Autodesk Inventor part; units mm, degrees
ref_plane "YZ Plane" through (0, 0, 0) normal (1, 0, 0) x (0, 1, 0)
ref_plane "XZ Plane" through (0, 0, 0) normal (0, 1, 0) x (-1, 0, 0)
ref_plane "XY Plane" through (0, 0, 0) normal (0, 0, 1) x (1, 0, 0)
sketch "Sketch1" plane through (0, 0, 0) normal (0, 0, 1) x (1, 0, 0)
  circle A0 centre (0, 0) radius 16.5
  arc A1 (-19.8431, 22.5) -> (-22.5, 19.8431) centre (0, 0) ccw
  arc A2 (22.5, 19.8431) -> (19.8431, 22.5) centre (0, 0) ccw
  arc A3 (-22.5, -19.8431) -> (-19.8431, -22.5) centre (0, 0) ccw
  arc A4 (19.8431, -22.5) -> (22.5, -19.8431) centre (0, 0) ccw
  line L0 (-22.5, -15) -> (-19.5, -12)
  line L1 (-19.5, 12) -> (-22.5, 15)
  line L2 (-15, -22.5) -> (-12, -19.5)
  line L3 (12, -19.5) -> (15, -22.5)
  line L4 (22.5, -15) -> (19.5, -12)
  line L5 (19.5, 12) -> (22.5, 15)
  line L6 (-22.5, -19.8431) -> (-22.5, -15)
  line L7 (-22.5, 15) -> (-22.5, 19.8431)
  line L8 (19.8431, -22.5) -> (15, -22.5)
  line L9 (-15, -22.5) -> (-19.8431, -22.5)
  line L10 (22.5, 19.8431) -> (22.5, 15)
  line L11 (22.5, -15) -> (22.5, -19.8431)
  line L12 (19.5, 4) -> (22.5, 4)
  line L13 (22.5, 4) -> (22.5, 2)
  line L14 (22.5, 2) -> (21.5, 2)
  line L15 (21.5, 2) -> (21.5, 3)
  line L16 (21.5, 3) -> (19.5, 3)
  line L17 (19.5, -4) -> (22.5, -4)
  line L18 (22.5, -4) -> (22.5, -2)
  line L19 (22.5, -2) -> (21.5, -2)
  line L20 (21.5, -2) -> (21.5, -3)
  line L21 (21.5, -3) -> (19.5, -3)
  line L22 (4, -19.5) -> (4, -22.5)
  line L23 (4, -22.5) -> (2, -22.5)
  line L24 (2, -22.5) -> (2, -21.5)
  line L25 (2, -21.5) -> (3, -21.5)
  line L26 (3, -21.5) -> (3, -19.5)
  line L27 (-3, -19.5) -> (-3, -21.5)
  line L28 (-3, -21.5) -> (-2, -21.5)
  line L29 (-2, -21.5) -> (-2, -22.5)
  line L30 (-2, -22.5) -> (-4, -22.5)
  line L31 (-4, -22.5) -> (-4, -19.5)
  line L32 (-19.5, -4) -> (-22.5, -4)
  line L33 (-22.5, -4) -> (-22.5, -2)
  line L34 (-22.5, -2) -> (-21.5, -2)
  line L35 (-21.5, -2) -> (-21.5, -3)
  line L36 (-21.5, -3) -> (-19.5, -3)
  line L37 (-19.5, 4) -> (-22.5, 4)
  line L38 (-22.5, 4) -> (-22.5, 2)
  line L39 (-22.5, 2) -> (-21.5, 2)
  line L40 (-21.5, 2) -> (-21.5, 3)
  line L41 (-21.5, 3) -> (-19.5, 3)
  line L42 (-12, -19.5) -> (-4, -19.5)
  line L43 (-3, -19.5) -> (3, -19.5)
  line L44 (4, -19.5) -> (12, -19.5)
  line L45 (-19.5, -12) -> (-19.5, -4)
  line L46 (-19.5, -3) -> (-19.5, 3)
  line L47 (-19.5, 4) -> (-19.5, 12)
  line L48 (19.5, -12) -> (19.5, -4)
  line L49 (19.5, -3) -> (19.5, 3)
  line L50 (19.5, 4) -> (19.5, 12)
  line L51 (-7.3937, 22.5) -> (-7, 27)
  line L52 (-7, 27) -> (7, 27)
  line L53 (7, 27) -> (7.3937, 22.5)
  arc A5 (-11.75, 20.9337) -> (-8.75, 20.9337) centre (-10.25, 19.5) ccw
  arc A6 (8.75, 20.9337) -> (11.75, 20.9337) centre (10.25, 19.5) ccw
  line L54 (-8.75, 20.9337) -> (-8.75, 22.5)
  line L55 (-11.75, 20.9337) -> (-11.75, 22.5)
  line L56 (8.75, 20.9337) -> (8.75, 22.5)
  line L57 (-19.8431, 22.5) -> (-11.75, 22.5)
  line L58 (-8.75, 22.5) -> (-7.3937, 22.5)
  line L59 (11.75, 20.9337) -> (11.75, 22.5)
  line L60 (7.3937, 22.5) -> (8.75, 22.5)
  line L61 (11.75, 22.5) -> (19.8431, 22.5)
  point P0 (-17, 17)
  point P1 (17, 17)
  point P2 (17, -17)
  point P3 (-17, -17)
  dimension "d0" = 33
  dimension "d7" = 30
  dimension "d8" = 30
  dimension "d9" = 30
  dimension "d10" = 30
  dimension "d14" = 30
  dimension "d15" = 15
  dimension "d16" = 15
  dimension "d19" = 22.5
  dimension "d22" = 8
  dimension "d23" = 4
  dimension "d24" = 2
  dimension "d25" = 1
  dimension "d27" = 1
  dimension "d28" = 3
  dimension "d29" = 4
  dimension "d30" = 8
  dimension "d31" = 19.5
  dimension "d32" = 19.5
  dimension "d33" = 19.5
  dimension "d34" = 17
  dimension "d35" = 17
  dimension "d36" = 17
  dimension "d37" = 17
  dimension "d38" = 14
  dimension "d39" = 7
  dimension "d40" = 14.7874
  dimension "d42" = 7.3937
  dimension "d47" = 4.15
  dimension "d48" = 20.5
  dimension "d49" = 10.25
  dimension "d51" = 1.5
  dimension "d56" = 1.5
  dimension "d57" = 3
  dimension "d58" = 22.5
  dimension "d59" = 4.5
extrude "SMC, 32MM" add sketch "Sketch1" along normal blind 25.4
hole "Hole1" at (-17, 17, 0) at (17, 17, 0) at (17, -17, 0) at (-17, -17, 0) direction (0, 0, 1) diameter 5.1054 end through all
equation "\"d16\" = d15"
equation "\"d27\" = d25"
equation "\"d30\" = d22"
equation "\"d11\" = d5"
equation "\"d12\" = d6"
properties part number "EXTRUSION, CYLINDER, ALUMINIUM, SMC, 32MM" material "Extrusion, Aluminum, SMC, 32 MM"
Check sheet for the modelled part. Datum: model origin and axes. Units: mm. A direction names the side the tool comes from. Coordinates: 2 decimals unless noted, no trailing zeros. Order: outer loops, then holes, each group sorted by start corner. A loop starts at its lowest first (then second) coordinate and runs counter-clockwise, first axis right, second up. Notation, with made-up numbers: (-15.5, 74) -> (42.5, 74) arc R8 cw to (42.5, 84) -> close; hole circle Ø7 at (29, -3). An arc over 180 degrees is marked (long way). Write item = value, one per line. Start each with the question number.
1) Cross-section at B-B (x = 0). Enter the section's corners in (y, z), then the cut area to 3 significant figures.
2) Cross-section at C-C (z = 17). State how many separate pieces and enclosed holes the cut face has, then the cut area to 3 significant figures.
3) Material ranges on L1, parallel to X at y = 17, z = 16.5; L2, parallel to Y at x = 0, z = 10.75, recorded low to high.
4) Go/stop test with flat-tipped pins: P1, Ø2.5, axis at x = -7.5, z = 18, coming from the -Y side; P2, Ø0.5, axis at x = -22, z = 13, coming from the -Y side; P3, Ø4, axis at y = -7.5, z = 18, coming from the -X side. Record where each tip stops, or that it passes through.
5) Cross-section at A-A (y = 0). Enter the section's corners in (x, z).
6) Mould release check, pull along Y, two halves, no side actions. Record for faces 1 (the cylindrical face through (14.848, -15.628, 12.878)), 2 (the flat face through (3, -22.5, 13)), 3 (the flat face through (19.5, 8, 13)), 4 (the cylindrical face through (-21.232, 21.195, 12.522)): +Y half, -Y half, draft (parallel to the pull), parting line (faces both ways), or undercut.
7) Access from +Z, -Z, +X, -X, +Y, -Y to the whole of each face (thin tool, end or side, straight path). Record for faces 5 (the flat face through (-13.5, -21, 12.5)), 6 (the flat face through (21, 13.5, 12.5)), 7 (the flat face through (-21, 13.5, 12.5)), 8 (the flat face through (8, 22.5, 13)).
Ans:
q1.outline = (-19.5, 0) -> (-16.5, 0) -> (-16.5, 25.4) -> (-19.5, 25.4) -> close; (16.5, 0) -> (27, 0) -> (27, 25.4) -> (16.5, 25.4) -> close
q1.area = 343 mm²
q2.separate_pieces = 1
q2.enclosed_holes = 5
q2.area = 886 mm²
q3.L1 = -22.5 to -19.55, -14.45 to 14.45, 19.55 to 22.5
q3.L2 = -19.5 to -16.5, 16.5 to 27
q4.P1 = -19.5
q4.P2 = -20.66
q4.P3 = -19.5
q5.outline = (-19.5, 0) -> (-16.5, 0) -> (-16.5, 25.4) -> (-19.5, 25.4) -> close; (16.5, 0) -> (19.5, 0) -> (19.5, 25.4) -> (16.5, 25.4) -> close
q6.face_1 = undercut
q6.face_2 = -Y half
q6.face_3 = undercut
q6.face_4 = +Y half
q7.face_5 = +Z, -Z, -Y
q7.face_6 = +Z, -Z, +X
q7.face_7 = +Z, -Z, -X
q7.face_8 = +Z, -Z, +X, +Y
